```python
from build123d import *

# Parameters (mm, degrees)
SKETCH1_R           = 2.25
BOSS_EXTRUDE1_DEPTH = 8.5


with BuildPart() as part:
    # Sketch1 → Boss-Extrude1 (new body)
    with BuildSketch(Plane(origin=(0, 0, 0), x_dir=(1, 0, 0), z_dir=(0, 1, 0))):
        with BuildLine():
            Line((-6, -3.5), (6, -3.5))
            ThreePointArc((6, -3.5), (9.5, 0), (6, 3.5))
            Line((6, 3.5), (-6, 3.5))
            ThreePointArc((-6, 3.5), (-9.5, 0), (-6, -3.5))
        make_face()
        with Locations((5, 0)):
            Circle(SKETCH1_R, mode=Mode.SUBTRACT)
        with Locations((-5, 0)):
            Circle(SKETCH1_R, mode=Mode.SUBTRACT)
    extrude(amount=BOSS_EXTRUDE1_DEPTH)


solid = part.part
```
Read the model definition and answer for the solid it produces. Units are mm, in the model's axes. Coordinates: 2 decimals unless noted, no trailing zeros. Write each loop counter-clockwise with the first axis right and the second up, starting at its lowest first coordinate (ties: lowest second). Pieces come first, ordered by that corner, then holes. Notation, with made-up numbers: (-26, 76.5) -> (-18, 76.5) arc R28 ccw to (-18, 97.5) -> close; hole circle Ø6 at (-38.5, -24.5). An arc over 180 degrees is marked (long way). Answer as a JSON object with one key per item and string values.
Q1. The part is cut by section D-D on x = -3.5. Give the vertices of the cut face in (y, z).
The answers:
{"outline": "(0, -3.5) -> (8.5, -3.5) -> (8.5, -1.68) -> (0, -1.68) -> close; (0, 1.68) -> (8.5, 1.68) -> (8.5, 3.5) -> (0, 3.5) -> close"}
Q2. The part is cut by section B-B on z = 0. Give the vertices of the cut face in (x, y).
The answers:
{"outline": "(-9.5, 0) -> (-7.25, 0) -> (-7.25, 8.5) -> (-9.5, 8.5) -> close; (-2.75, 0) -> (2.75, 0) -> (2.75, 8.5) -> (-2.75, 8.5) -> close; (7.25, 0) -> (9.5, 0) -> (9.5, 8.5) -> (7.25, 8.5) -> close"}
Q3. The part is cut by section A-A on x = 5. Give the vertices of the cut face in (y, z).
The answers:
{"outline": "(0, -3.5) -> (8.5, -3.5) -> (8.5, -2.25) -> (0, -2.25) -> close; (0, 2.25) -> (8.5, 2.25) -> (8.5, 3.5) -> (0, 3.5) -> close"}
Q4. The part is cut by section C-C on y = 7. Give the vertices of the cut face in (x, z).
The answers:
{"outline": "(-6, -3.5) -> (6, -3.5) arc R3.5 ccw to (6, 3.5) -> (-6, 3.5) arc R3.5 ccw to start; hole circle Ø4.5 at (-5, 0); hole circle Ø4.5 at (5, 0)"}
Q5. Consider line 1 (X direction, y = 4, z = 0); line 2 (X direction, y = 4.25, z = -1.75); line 3 (Z direction, x = 5, y = 6). Determine where each line is inside the solid, lowest interval first. Write a range as [from, to].
The answers:
{"line 1": "x = [-9.5, -7.25], [-2.75, 2.75], [7.25, 9.5]", "line 2": "x = [-9.03, -6.41], [-3.59, 3.59], [6.41, 9.03]", "line 3": "z = [-3.5, -2.25], [2.25, 3.5]"}
Q6. Determine the mould class of faces 1 (the cylindrical face through (-2.854, 4.19, -0.676)), 2 (the flat face through (0, 4, 3.5)), 3 (the cylindrical face through (-9.5, 4.2, -0.1)), 4 (the flat face through (0, 0, 0)) for opening direction Z: pulls with the +Z half, pulls with the -Z half, needs draft (parallel to the pull), parting line crosses it, or undercut.
The answers:
{"face 1": "undercut", "face 2": "pulls with the +Z half", "face 3": "parting line crosses it", "face 4": "needs draft"}
